The figure shows three views and two pictorial views of one solid part (mm, origin at its lowest corner). Answer the questions. A direction names the side the tool comes from. Coordinates: 2 decimals unless noted, no trailing zeros. Loops run counter-clockwise (first coordinate to the right, second up) from the corner with the lowest first, then second, coordinate; pieces in that order, holes last. Notation, with made-up numbers: (62.25, -34.5) - (102.25, -34.5) arc R20 ccw to (102.25, 1.5) - close; hole circle Ø9 at (61.25, 60). An arc over 180 degrees is marked (long way). Return JSON: item names as keys, results as strings. Group by question number.
1. Section B-B (z = 7.5) is taken. Write down the section's boundary in (x, y).
2. Find the intervals of material crossed by line 1 along Y through (x, z) = (8.5, 2.5); line 2 along X through (y, z) = (2.75, 7.25); line 3 along Y through (x, z) = (6.5, 11.5), in increasing order.
3. Which of the six approach directions +Z, -Z, +X, -X, +Y, -Y give full straight-line access (tool end or side, diameter ignored) to the marked faces 1, 2 and 3?
4. Section A-A (x = 7.5) is taken. Write down the section's boundary in (y, z).
5. Each of these flat-tipped pins is pushed along its axis until it touches: P1, Ø1.5, axis at x = 13, y = 8.5, coming from the +Z side; P2, Ø3.5, axis at y = 1.5, z = 7.5, coming from the +X side; P3, Ø0.9, axis at y = 2, z = 8, coming from the -X side. Where does it stop, or does it pass through?
6. Section C-C (y = 8.75) is taken. Write down the section's boundary in (x, z).
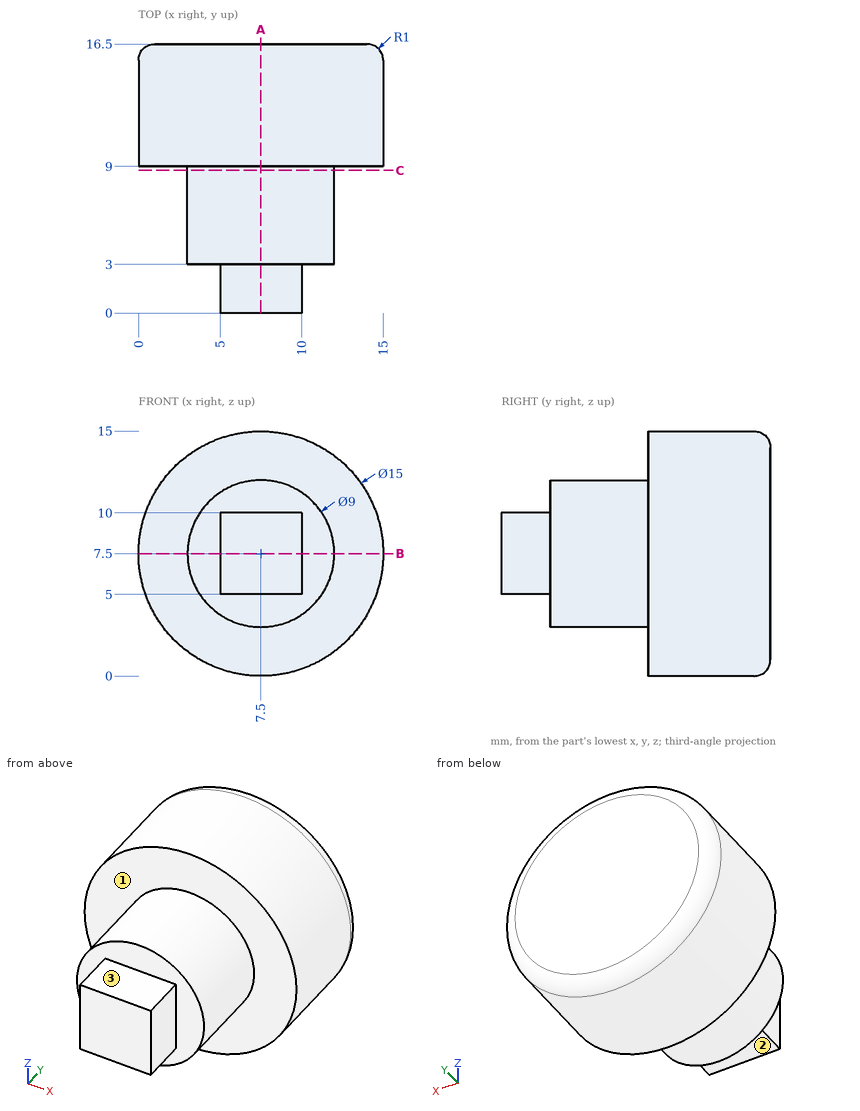
The answers:
{
 "1": {"outline": "(0, 9) - (3, 9) - (3, 3) - (5, 3) - (5, 0) - (10, 0) - (10, 3) - (12, 3) - (12, 9) - (15, 9) - (15, 15.5) arc R1 ccw to (14, 16.5) - (1, 16.5) arc R1 ccw to (0, 15.5) - close"},
 "2": {"line 1": "y = 9 to 16.5", "line 2": "x = 5 to 10", "line 3": "y = 3 to 16.5"},
 "3": {"face 1": "-Y", "face 2": "-Z, +X, -X, -Y", "face 3": "+Z, +X, -X, -Y"},
 "4": {"outline": "(0, 5) - (3, 5) - (3, 3) - (9, 3) - (9, 0) - (15.5, 0) arc R1 ccw to (16.5, 1) - (16.5, 14) arc R1 ccw to (15.5, 15) - (9, 15) - (9, 12) - (3, 12) - (3, 10) - (0, 10) - close"},
 "5": {"P1": "stops at z = 13.14", "P2": "stops at x = 12", "P3": "stops at x = 5"},
 "6": {"outline": "circle Ø9 at (7.5, 7.5)"}
}
